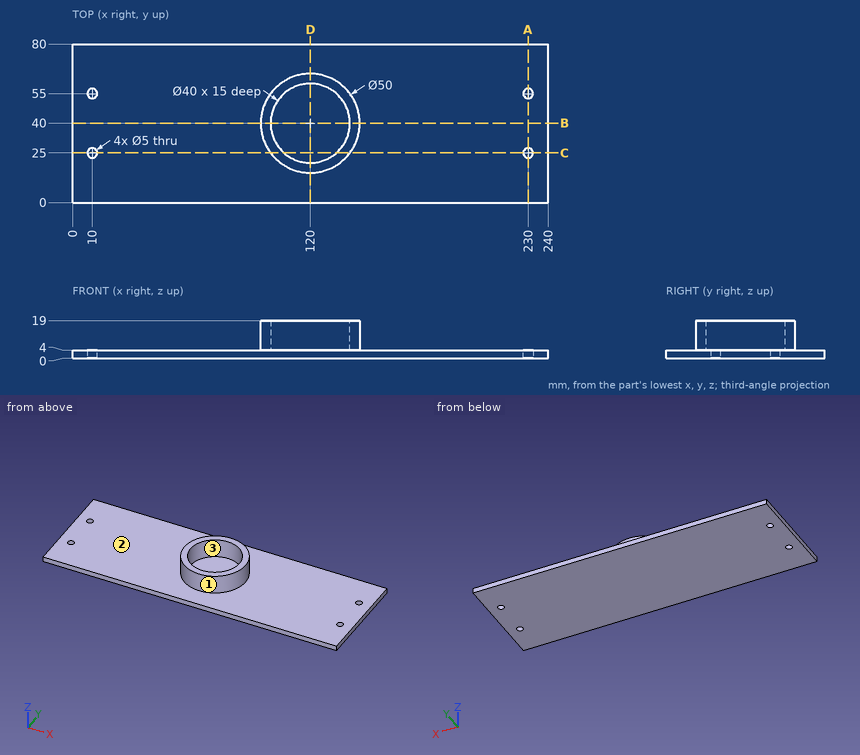
Answer from the drawing. Dimensions are ordinates in mm from the lowest x, y and z of the part. Round coordinates to 2 decimals unless told otherwise and drop trailing zeros. Loops run counter-clockwise (first coordinate to the right, second up) from the corner with the lowest first, then second, coordinate; pieces in that order, holes last.
Q1. Section D-D on x = 120 is taken. Write down the section's boundary in (y, z), and give its area (3 significant figures).
Q2. Section A-A on x = 230 is taken. Write down the section's boundary in (y, z), and give its area (3 significant figures).
Q3. Section B-B on y = 40 is taken. Write down the section's boundary in (x, z).
Q4. Each of these flat-tipped pins is pushed along its axis until it touches: pin 1 (20 mm diameter, centred on x = 110.5, y = 43, fed in from +Z); pin 2 (4 mm diameter, centred on x = 10, y = 55, fed in from +Z). Where does it stop, or does it pass through?
Q5. Consider probe 1 along Y at (x, z) = (10, 1.1); probe 2 along Z at (x, y) = (175.5, 28); probe 3 along Y at (x, z) = (120, 15). Determine where each line is inside the solid, lowest interval first.
Q6. Section C-C on y = 25 is taken. Write down the section's boundary in (x, z), and give its area (3 significant figures).
Q7. Determine the mould class of the marked faces 1, 2 and 3 for opening direction X: released by +X, released by -X, zero draft, split by the parting line, or undercut.
Output:
1. outline: (0, 0) - (80, 0) - (80, 4) - (65, 4) - (65, 19) - (60, 19) - (60, 4) - (20, 4) - (20, 19) - (15, 19) - (15, 4) - (0, 4) - close
1. area: 470 mm2
2. outline: (0, 0) - (22.5, 0) - (22.5, 4) - (0, 4) - close; (27.5, 0) - (52.5, 0) - (52.5, 4) - (27.5, 4) - close; (57.5, 0) - (80, 0) - (80, 4) - (57.5, 4) - close
2. area: 280 mm2
3. outline: (0, 0) - (240, 0) - (240, 4) - (145, 4) - (145, 19) - (140, 19) - (140, 4) - (100, 4) - (100, 19) - (95, 19) - (95, 4) - (0, 4) - close
4. pin 1: stops at z = 4
4. pin 2: passes through
5. probe 1: y = 0 to 22.5, 27.5 to 52.5, 57.5 to 80
5. probe 2: z = 0 to 4
5. probe 3: y = 15 to 20, 60 to 65
6. outline: (0, 0) - (7.5, 0) - (7.5, 4) - (0, 4) - close; (12.5, 0) - (227.5, 0) - (227.5, 4) - (140, 4) - (140, 19) - (133.23, 19) - (133.23, 4) - (106.77, 4) - (106.77, 19) - (100, 19) - (100, 4) - (12.5, 4) - close; (232.5, 0) - (240, 0) - (240, 4) - (232.5, 4) - close
6. area: 1,120 mm2
7. face 1: split by the parting line
7. face 2: zero draft
7. face 3: undercut
